For this review, use the dimensioned drawing (mm, ordinates from the lowest corner) and the shaded views. Round coordinates to 2 decimals unless told otherwise and drop trailing zeros. Write each loop counter-clockwise with the first axis right and the second up, starting at its lowest first coordinate (ties: lowest second). Pieces come first, ordered by that corner, then holes. Notation, with made-up numbers: M 49.25,-39.75 L 99.25,-39.75 A29 ccw 99.25,-1.75 Z; hole C -35,-14.75 d10. An arc over 180 degrees is marked long. One line per question, with ' | ' between items. Start each with the question number.
Item 1: Add section B-B, the plane y = 18. State the section outline as (x, z) points.
Item 2: Insertion check: pin 1 Ø1 at (x, z) = (12, 7) entering from +Y; pin 2 Ø1 at (x, z) = (3, 8) entering from +Y; pin 3 Ø6 at (x, z) = (13.5, 6) entering from +Y. Each pin has a flat end and moves straight along its axis. Give the tip position at first contact, or say it passes through.
Item 3: Add section A-A, the plane z = 4. State the section outline as (x, y) points.
Item 4: Add section C-C, the plane x = 8.5. State the section outline as (y, z) points, and give its area (3 significant figures).
Item 5: For L1, parallel to X at y = 21, z = 5; L2, parallel to Y at x = 11, z = 9.5; L3, parallel to Y at x = 8.25, z = 0.5, list the stretches that pass through material, from the lowest coordinate up.
Item 6: Add section D-D, the plane x = 16. State the section outline as (y, z) points, and give its area (3 significant figures).
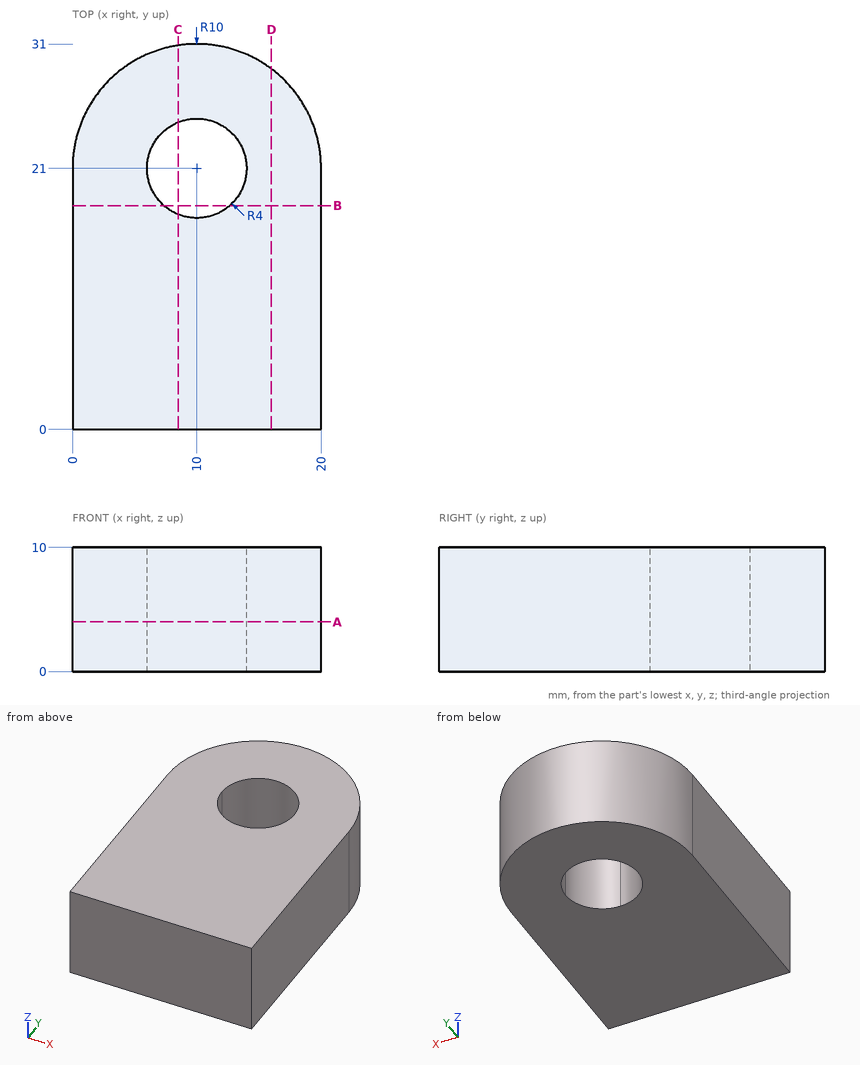
Computed values:
1) outline: M 0,0 L 7.35,0 L 7.35,10 L 0,10 Z; M 12.65,0 L 20,0 L 20,10 L 12.65,10 Z
2) pin 1: stops at y = 30.89 | pin 2: stops at y = 28.6 | pin 3: stops at y = 30.99
3) outline: M 0,0 L 20,0 L 20,21 A10 ccw 0,21 Z; hole C 10,21 d8
4) outline: M 0,0 L 17.29,0 L 17.29,10 L 0,10 Z; M 24.71,0 L 30.89,0 L 30.89,10 L 24.71,10 Z | area: 235 mm^2
5) L1: x = 0 to 6, 14 to 20 | L2: y = 0 to 17.13, 24.87 to 30.95 | L3: y = 0 to 17.4, 24.6 to 30.85
6) outline: M 0,0 L 29,0 L 29,10 L 0,10 Z | area: 290 mm^2
